Input: part model. Units: mm. Frame: model coordinates. A direction names the side the tool comes from. Round coordinates to 2 decimals unless told otherwise and drop trailing zeros. Order: outer loops, then holes, each group sorted by start corner. A loop starts at its lowest first (then second) coordinate and runs counter-clockwise, first axis right, second up. Notation, with made-up numbers: (9, 85) - (29, 85) arc R34 ccw to (29, 122) - close; hole circle Ø5 at (-15, -9.75). An arc over 180 degrees is marked (long way). One line per item, written item: value. Start each with the question number.
from build123d import *

# Parameters (mm, degrees)
SKETCH_1_R                = 62.5
EXTRUDE_1_DEPTH           = 10
SKETCH_2_R                = 50
CUT_EXTRUDE_1_DEPTH       = 89.952234373
SKETCH_3_R                = 52.5
CUT_EXTRUDE_2_DEPTH       = 5
HOLE_WIZARD_9_D           = 4.5
HOLE_WIZARD_9_CBORE_D     = 10
HOLE_WIZARD_9_CBORE_DEPTH = 3
PATTERN_CIRCULAR_1_COUNT  = 12


with BuildPart() as part:
    # 草图1 → 凸台-拉伸1 (new body)
    with BuildSketch(Plane.XY):
        Circle(SKETCH_1_R)
    extrude(amount=EXTRUDE_1_DEPTH)

    # 草图2 → 切除-拉伸1 (cut, through all)
    with BuildSketch(Plane.XY.offset(10)):
        Circle(SKETCH_2_R)
    extrude(amount=-CUT_EXTRUDE_1_DEPTH, mode=Mode.SUBTRACT)

    # 草图3 → 切除-拉伸2 (cut)
    with BuildSketch(Plane.XY.offset(10)):
        Circle(SKETCH_3_R)
    extrude(amount=-CUT_EXTRUDE_2_DEPTH, mode=Mode.SUBTRACT)

    # 打孔尺寸(%根据六角头螺)栓 全螺纹的类型9 (through all)
    with Locations(Plane(origin=(0, 0, 0), x_dir=(-1, 0, 0), z_dir=(0, 0, -1))):
        with Locations((0, 57)):
            hole_wizard_9 = CounterBoreHole(HOLE_WIZARD_9_D / 2, HOLE_WIZARD_9_CBORE_D / 2, HOLE_WIZARD_9_CBORE_DEPTH)

    # 阵列(圆周)1: 打孔尺寸(%根据六角头螺)栓 全螺纹的类型9 ×12 about axis
    pattern_circular_1_axis = Axis((0, 0, 0), (0, 0, 1))
    for i in range(1, PATTERN_CIRCULAR_1_COUNT):
        add(hole_wizard_9.rotate(pattern_circular_1_axis, i * 360 / PATTERN_CIRCULAR_1_COUNT), mode=Mode.SUBTRACT)


solid = part.part
Item 1: Reachability of faces 1 (the face through (61.957, -0.651, 1.479)), 2 (the face through (-0.29, 59.23, 6.55)) from +Z, -Z, +X, -X, +Y, -Y: full face, straight path, thin tool, end or side. Return the list, or none.
Item 2: Section query C-C on y = -16. Return loops of the section in (x, z).
Item 3: Line query: L1, parallel to Y at x = 0, z = 6; L2, parallel to Y at x = -33, z = 1.75; L3, parallel to Z at x = 50, y = 31.5. Output: solid intervals per line, ascending.
Item 4: Section query D-D on z = 8.5. Give the number of separate pieces and of enclosed holes in the cut face, and give its area (3 significant figures).
Item 5: Section query A-A on x = 0. Return loops of the section in (y, z), and give its area (3 significant figures).
Item 6: First-contact query: pin 1 Ø3 at (x, y) = (0.5, -55) entering from -Z; pin 2 Ø1 at (x, z) = (26.5, 3.5) entering from +Y; pin 3 Ø1.5 at (y, z) = (5.5, 1.5) entering from +X. Flat tips, straight axial feed; report the tip coordinate or a pass-through.
Geometry results:
1. face 1: -Z
1. face 2: +Z, -Z
2. outline: (-60.42, 0) - (-47.37, 0) - (-47.37, 5) - (-50, 5) - (-50, 10) - (-60.42, 10) - close; (47.37, 0) - (60.42, 0) - (60.42, 10) - (50, 10) - (50, 5) - (47.37, 5) - close
3. L1: y = -62.5 to -59.25, -54.75 to -52.5, 52.5 to 54.75, 59.25 to 62.5
3. L2: y = -53.08 to -51.54, -47.18 to -37.56, 37.56 to 47.18, 51.54 to 53.08
3. L3: z = 3 to 10
4. separate pieces: 1
4. enclosed holes: 13
4. area: 3,420 mm^2
5. outline: (-62.5, 0) - (-62, 0) - (-62, 3) - (-59.25, 3) - (-59.25, 10) - (-62.5, 10) - close; (-54.75, 3) - (-52, 3) - (-52, 0) - (-50, 0) - (-50, 5) - (-52.5, 5) - (-52.5, 10) - (-54.75, 10) - close; (50, 0) - (52, 0) - (52, 3) - (54.75, 3) - (54.75, 10) - (52.5, 10) - (52.5, 5) - (50, 5) - close; (59.25, 3) - (62, 3) - (62, 0) - (62.5, 0) - (62.5, 10) - (59.25, 10) - close
5. area: 102 mm^2
6. pin 1: stops at z = 3
6. pin 2: stops at y = 56.84
6. pin 3: stops at x = 62.32
